from build123d import *

# Parameters (mm, degrees)
SKETCH1_W           = 50
SKETCH1_H           = 7
BOSS_EXTRUDE1_DEPTH = 1
SKETCH2_R           = 1.5
CUT_EXTRUDE1_DEPTH  = 39.281330669
LPATTERN2_COUNT     = 5
LPATTERN2_PITCH     = 10


with BuildPart() as part:
    # Sketch1 → Boss-Extrude1 (new body)
    with BuildSketch(Plane(origin=(0, 0, 0), x_dir=(1, 0, 0), z_dir=(0, 1, 0))):
        with Locations((-8.6, 14.816666667)):
            Rectangle(SKETCH1_W, SKETCH1_H)
    extrude(amount=BOSS_EXTRUDE1_DEPTH)

    # Sketch2 → Cut-Extrude1 (cut, through all)
    with BuildSketch(Plane(origin=(0, 1, 0), x_dir=(1, 0, 0), z_dir=(0, 1, 0))):
        with Locations(Location((-28.000173189, 14.816666667, 0), (0, 0, 270))):
            Circle(SKETCH2_R)
    cut_extrude1 = extrude(amount=-CUT_EXTRUDE1_DEPTH, mode=Mode.SUBTRACT)

    # LPattern2: Cut-Extrude1 ×5
    with Locations(*[(i * LPATTERN2_PITCH, 0, 0) for i in range(1, LPATTERN2_COUNT)]):
        add(cut_extrude1, mode=Mode.SUBTRACT)


solid = part.part
Can you work these out from the model? Positions are in its coordinate system, mm. Give positions to 0.01 mm unless a question says otherwise; leave off trailing zeros. Order: outer loops, then holes, each group sorted by start corner. A loop starts at its lowest first (then second) coordinate and runs counter-clockwise, first axis right, second up. Notation, with made-up numbers: M 58,68.25 L 106,68.25 A24 ccw 106,80.25 Z; hole C 8.5,43.5 d8. An arc over 180 degrees is marked long. Use a Markdown table: item, result. Add a question column.
Item 1: Suppose I cut it at B-B (x = -27.5). List the corners of the cut face in (y, z) for me, then the cut area to 3 significant figures.
Item 2: Suppose I cut it at A-A (z = -14). List the corners of the cut face in (x, y) for me, then the cut area to 3 significant figures.
Item 3: Suppose I cut it at C-C (y = 0.55). List the corners of the cut face in (x, z) for me, then the cut area to 3 significant figures.
Item 4: Suppose I cut it at D-D (x = -19). List the corners of the cut face in (y, z) for me.
Item 5: We'd pull the mould along X, two halves only. Please class faces 1 (the cylindrical face through (-29.33, 0.51, -14.12)), 2 (the flat face through (-9, 0.5, -18.317)), 3 (the flat face through (-33.6, 0.5, -14.8)): +X half, -X half, draft (parallel to the pull), parting line (faces both ways), or undercut.
Item 6: If I drill on L1, parallel to Z at x = -18, y = 0.7; L2, parallel to X at y = 0.3, z = -14.5; L3, parallel to X at y = 0.6, z = -15.5, over which ranges is the centre line in solid material (lowest first)? Write a range as [from, to].
Answer sheet:
| question | item | result |
|---|---|---|
| 1 | outline | M 0,-18.32 L 1,-18.32 L 1,-16.23 L 0,-16.23 Z; M 0,-13.4 L 1,-13.4 L 1,-11.32 L 0,-11.32 Z |
| 1 | area | 4.17 mm² |
| 2 | outline | M -33.6,0 L -29.26,0 L -29.26,1 L -33.6,1 Z; M -26.74,0 L -19.26,0 L -19.26,1 L -26.74,1 Z; M -16.74,0 L -9.26,0 L -9.26,1 L -16.74,1 Z; M -6.74,0 L 0.74,0 L 0.74,1 L -6.74,1 Z; M 3.26,0 L 10.74,0 L 10.74,1 L 3.26,1 Z; M 13.26,0 L 16.4,0 L 16.4,1 L 13.26,1 Z |
| 2 | area | 37.4 mm² |
| 3 | outline | M -33.6,-18.32 L 16.4,-18.32 L 16.4,-11.32 L -33.6,-11.32 Z; hole C -28,-14.82 d3; hole C -18,-14.82 d3; hole C -8,-14.82 d3; hole C 2,-14.82 d3; hole C 12,-14.82 d3 |
| 3 | area | 315 mm² |
| 4 | outline | M 0,-18.32 L 1,-18.32 L 1,-15.93 L 0,-15.93 Z; M 0,-13.7 L 1,-13.7 L 1,-11.32 L 0,-11.32 Z |
| 5 | face 1 | undercut |
| 5 | face 2 | draft |
| 5 | face 3 | -X half |
| 6 | L1 | z = [-18.32, -16.32], [-13.32, -11.32] |
| 6 | L2 | x = [-33.6, -29.47], [-26.53, -19.47], [-16.53, -9.47], [-6.53, 0.53], [3.47, 10.53], [13.47, 16.4] |
| 6 | L3 | x = [-33.6, -29.34], [-26.66, -19.34], [-16.66, -9.34], [-6.66, 0.66], [3.34, 10.66], [13.34, 16.4] |
